Can you work these out from the model? Positions are in its coordinate system, mm. A direction names the side the tool comes from. Coordinates: 2 decimals unless noted, no trailing zeros. Order: outer loops, then holes, each group sorted by start corner. A loop starts at its lowest first (then second) coordinate and runs counter-clockwise, first axis right, second up. Notation, with made-up numbers: (12, 3.25) - (56, 3.25) arc R37 ccw to (56, 41.25) - close; hole circle Ø11 at (24.5, 65.25). An arc over 180 degrees is marked (long way). Use a Markdown table: item, result. Add a question column.
(1) I want a section at B-B (y = 5). List the corners of the cut face in (x, z) for me.
(2) I want a section at A-A (z = 0). List the corners of the cut face in (x, y) for me.
(3) If I drill on L1, parallel to Y at x = 7.5, z = 8.5; L2, parallel to X at y = 34.5, z = -0.25; L3, parallel to Y at x = 7.5, z = 3.75, over which ranges is the centre line in solid material (lowest first)? Write a range as [from, to].
(4) On a 3-axis mill with a long thin cutter (end or side, diameter ignored), from which of +Z, -Z, +X, -X, +Y, -Y can I reach the whole of each face in a straight line? I mean faces 1 (the flat face through (-12, 9.5, -6)), 2 (the flat face through (-7.2, 70.5, -2.6)), 3 (the flat face through (-11, 9.5, 8)), 4 (the flat face through (-5.52, 4.68, 11.77)), 5 (the flat face through (12.954, 4.684, -1.1)). Say none if no direction works.
(5) For pin 1 Ø3 at (y, z) = (65.5, -7) entering from +X; pin 2 Ø5 at (x, z) = (-9, -6) entering from +Y; pin 3 Ø8 at (x, y) = (9, 33) entering from -Z, each with a flat end and sliding along its axis, tell me the tip position at first contact or that it passes through.
(6) I want a section at C-C (x = -2.5). List the corners of the cut face in (y, z) for me.
(7) I want a section at D-D (y = 67). List the corners of the cut face in (x, z) for me, and give its area (3 significant figures).
```python
from build123d import *

# Parameters (mm, degrees)
EXTRUDE_1_DEPTH = 9.5
SKETCH_2_R      = 13
EXTRUDE_2_DEPTH = 7
SKETCH_3_R      = 11.05
EXTRUDE_3_DEPTH = 54
SKETCH_4_R      = 7.5
EXTRUDE_4_DEPTH = 3


with BuildPart() as part:
    # 草图1 → 凸台-拉伸1 (new body)
    with BuildSketch(Plane(origin=(0, 0, 0), x_dir=(1, 0, 0), z_dir=(0, 1, 0))):
        Polygon((13.639438395, -6.268895724), (12.248742148, 8.677652282), (-1.390696247, 14.946548006), (-13.639438395, 6.268895724), (-12.248742148, -8.677652282), (1.390696247, -14.946548006), align=None)
    extrude(amount=EXTRUDE_1_DEPTH)

    # 草图2 → 凸台-拉伸2 (add)
    with BuildSketch(Plane(origin=(0, 9.5, 0), x_dir=(1, 0, 0), z_dir=(0, 1, 0))):
        with Locations(Location((0, 0, 0), (0, 0, 65.31576064))):
            Circle(SKETCH_2_R)
    extrude(amount=EXTRUDE_2_DEPTH)

    # 草图3 → 凸台-拉伸3 (add)
    with BuildSketch(Plane(origin=(0, 16.5, 0), x_dir=(1, 0, 0), z_dir=(0, 1, 0))):
        with Locations(Location((0, 0, 0), (0, 0, 270))):
            Circle(SKETCH_3_R)
    extrude(amount=EXTRUDE_3_DEPTH)

    # 草图4 → 凸台-拉伸4 (add)
    with BuildSketch(Plane(origin=(0, 70.5, 0), x_dir=(1, 0, 0), z_dir=(0, 1, 0))):
        with Locations(Location((0, 0, 0), (0, 0, 270))):
            Circle(SKETCH_4_R)
    extrude(amount=EXTRUDE_4_DEPTH)


solid = part.part
```
Answers follow:
| question | item | result |
|---|---|---|
| 1 | outline | (-13.64, -6.27) - (-1.39, -14.95) - (12.25, -8.68) - (13.64, 6.27) - (1.39, 14.95) - (-12.25, 8.68) - close |
| 2 | outline | (-13.06, 0) - (13.06, 0) - (13.06, 9.5) - (13, 9.5) - (13, 16.5) - (11.05, 16.5) - (11.05, 70.5) - (7.5, 70.5) - (7.5, 73.5) - (-7.5, 73.5) - (-7.5, 70.5) - (-11.05, 70.5) - (-11.05, 16.5) - (-13, 16.5) - (-13, 9.5) - (-13.06, 9.5) - close |
| 3 | L1 | y = [0, 16.5] |
| 3 | L2 | x = [-11.05, 11.05] |
| 3 | L3 | y = [0, 70.5] |
| 4 | face 1 | -Z, -X, +Y |
| 4 | face 2 | +Y |
| 4 | face 3 | +Z, -X, +Y |
| 4 | face 4 | +Z, -X, +Y, -Y |
| 4 | face 5 | -Z, +X, +Y, -Y |
| 5 | pin 1 | stops at x = 9.58 |
| 5 | pin 2 | stops at y = 70.5 |
| 5 | pin 3 | stops at z = -9.85 |
| 6 | outline | (0, -14.16) - (9.5, -14.16) - (9.5, -12.76) - (16.5, -12.76) - (16.5, -10.76) - (70.5, -10.76) - (70.5, -7.07) - (73.5, -7.07) - (73.5, 7.07) - (70.5, 7.07) - (70.5, 10.76) - (16.5, 10.76) - (16.5, 12.76) - (9.5, 12.76) - (9.5, 13.16) - (0, 13.16) - close |
| 7 | outline | circle Ø22.1 at (0, 0) |
| 7 | area | 384 mm² |
